The listing builds one solid part. Answer for the finished solid, in the listing's coordinates (mm). A direction names the side the tool comes from. Give positions to 0.01 mm unless a question says otherwise; leave off trailing zeros. Loops run counter-clockwise (first coordinate to the right, second up) from the corner with the lowest first, then second, coordinate; pieces in that order, holes last. Notation, with made-up numbers: (-9.75, 60.5) - (31.25, 60.5) arc R30 cw to (31.25, 98.5) - close; hole circle Ø5 at (71, 16.5). An arc over 180 degrees is marked (long way). Write item = value, one per line. Start each with the question number.
1) The part is cut by section C-C on x = 349. Write down the section's boundary in (y, z), plus the area to 3 significant figures.
2) Consider probe 1 along Z at (x, y) = (334.5, 76); probe 2 along X at (y, z) = (90, -143.5); probe 3 along Y at (x, z) = (301, -161.5). Determine where each line is inside the solid, lowest interval first.
3) The part is cut by section A-A on y = 33. Write down the section's boundary in (x, z).
4) A flat-ended cylindrical pin translates along its axis: P1, Ø1.5, axis at x = 126.5, z = -179.5, coming from the +Y side. Find the tip coordinate at first contact, or state that the pin passes through.
5) The part is cut by section B-B on z = -152. Write down the section's boundary in (x, y), plus the area to 3 significant figures.
6) Which of the six approach directions +Z, -Z, +X, -X, +Y, -Y give full straight-line access (tool end or side, diameter ignored) to faces 1 (the flat face through (0, 50, -103)), 2 (the flat face through (257, 61, -19.05))?
7) The mould has two halves that part along Z. Classify faces 3 (the flat face through (250, 50, 0)), 4 (the flat face through (258, 0, -100)), 5 (the flat face through (488.95, 61, -103)): +Z half, -Z half, draft (parallel to the pull), parting line (faces both ways), or undercut.
Autodesk Inventor part; units mm, degrees
ref_plane "YZ Plane" through (0, 0, 0) normal (1, 0, 0) x (0, 1, 0)
ref_plane "XZ Plane" through (0, 0, 0) normal (0, 1, 0) x (-1, 0, 0)
ref_plane "XY Plane" through (0, 0, 0) normal (0, 0, 1) x (1, 0, 0)
sketch "Sketch4" plane through (0, 0, 0) normal (0, 1, 0) x (-1, 0, 0)
  line L0 (0, 0) -> (-508, 0)
  line L1 (-508, 0) -> (-508, -203.2)
  line L2 (-508, -203.2) -> (0, -203.2)
  line L3 (0, -203.2) -> (0, 0)
  line L4 (0, 0) -> (-19.05, 0)
  dimension "d14" = 508
  dimension "d15" = 203.2
  dimension "d16" = 19.05
extrude "Extrusion3" add sketch "Sketch4" along normal blind 101.6
sketch "Sketch5" plane through (0, 101.6, 0) normal (0, 1, 0) x (1, 0, 0)
  line L0 (0, 0) -> (508, 0)
  line L1 (508, 203.2) -> (0, 203.2)
  line L2 (0, 0) -> (19.05, 0)
  line L3 (19.05, 19.05) -> (19.05, 184.15)
  line L4 (19.05, 184.15) -> (488.95, 184.15)
  line L5 (488.95, 184.15) -> (488.95, 19.05)
  line L6 (488.95, 19.05) -> (19.05, 19.05)
  dimension "d21" = 165.1
  dimension "d22" = 469.9
  dimension "d23" = 165.1
extrude "Extrusion4" cut sketch "Sketch5" against normal blind 82.55
fillet "Fillet5" radius 6.35 1 edges at (488.95, 60.325, -184.15)
fillet "Fillet6" radius 6.35 1 edges at (19.05, 60.325, -184.15)
fillet "Fillet7" radius 6.35 1 edges at (19.05, 60.325, -19.05)
fillet "Fillet8" radius 6.35 1 edges at (488.95, 60.325, -19.05)
properties part number "Box" material "Acetal Resin, Black"
Answer below:
q1.outline = (0, -203.2) - (101.6, -203.2) - (101.6, -184.15) - (19.05, -184.15) - (19.05, -19.05) - (101.6, -19.05) - (101.6, 0) - (0, 0) - close
q1.area = 7,020 mm2
q2.probe_1 = -203.2 to -184.15, -19.05 to 0
q2.probe_2 = 0 to 19.05, 488.95 to 508
q2.probe_3 = 0 to 19.05
q3.outline = (0, -203.2) - (508, -203.2) - (508, 0) - (0, 0) - close; hole (19.05, -177.8) arc R6.35 ccw to (25.4, -184.15) - (482.6, -184.15) arc R6.35 ccw to (488.95, -177.8) - (488.95, -25.4) arc R6.35 ccw to (482.6, -19.05) - (25.4, -19.05) arc R6.35 ccw to (19.05, -25.4) - close
q4.P1 = 19.05
q5.outline = (0, 0) - (508, 0) - (508, 101.6) - (488.95, 101.6) - (488.95, 19.05) - (19.05, 19.05) - (19.05, 101.6) - (0, 101.6) - close
q5.area = 12,800 mm2
q6.face_1 = +Z, -Z, -X, +Y, -Y
q6.face_2 = +Y
q7.face_3 = +Z half
q7.face_4 = draft
q7.face_5 = undercut
